Here's the drawing with two shaded views (mm, measured from the low corner). I have some questions. A direction names the side the tool comes from. Round coordinates to 2 decimals unless told otherwise and drop trailing zeros. Write each loop counter-clockwise with the first axis right and the second up, starting at its lowest first coordinate (ties: lowest second). Pieces come first, ordered by that corner, then holes. Notation, with made-up numbers: M 89,54.25 L 108,54.25 A19 cw 108,83.25 Z; hole C 73,3.5 d2. An arc over 180 degrees is marked long. Write item = value, one per line. Start each with the question number.
(1) I want a section at D-D (z = 4). Give the number of separate pieces and of enclosed holes in the cut face, and give its area (3 significant figures).
(2) I want a section at B-B (x = 69.85). List the corners of the cut face in (y, z) for me (1 decimal).
(3) Will these pins go through, and if not, where does the flat tip stop? pin 1 Ø1 at (y, z) = (9, 3) entering from +X; pin 2 Ø4.5 at (x, z) = (31.5, 1.5) entering from -Y (1 decimal); pin 3 Ø4.5 at (x, z) = (38, 2) entering from +Y (1 decimal); pin 4 Ø3 at (x, z) = (69.85, 8.89) entering from -Y.
(4) I need wall thicknesses on line 1 along Y through (x, z) = (25.4, 6.5); line 2 along X through (y, z) = (9.75, 8.75); line 3 along Y through (x, z) = (25.4, 4.25) (1 decimal). Which ranges of each line are inside material? Lowest first, please.
(5) I want a section at A-A (z = 8.89). List the corners of the cut face in (x, y) for me, and give its area (3 significant figures).
(6) On a 3-axis mill with a long thin cutter (end or side, diameter ignored), from which of +Z, -Z, +X, -X, +Y, -Y can I reach the whole of each face in a straight line? I mean the marked faces 1, 2 and 3. Say none if no direction works.
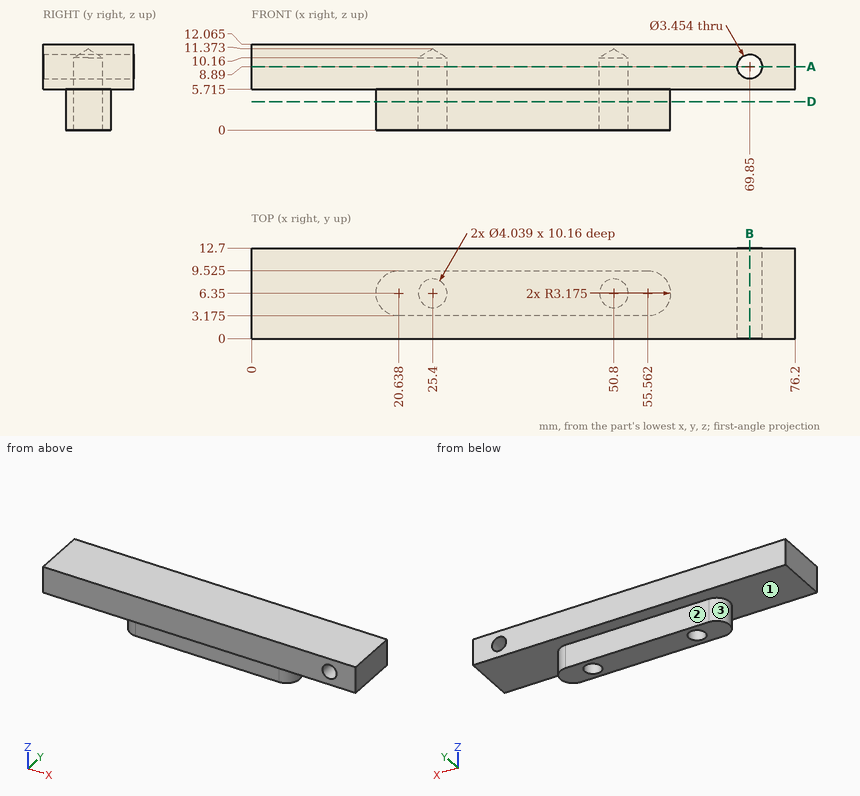
Returned:
q1.separate_pieces = 1
q1.enclosed_holes = 2
q1.area = 228 mm²
q2.outline = M 0,5.7 L 12.7,5.7 L 12.7,7.2 L 0,7.2 Z; M 0,10.6 L 12.7,10.6 L 12.7,12.1 L 0,12.1 Z
q3.pin_1 = 57.9
q3.pin_2 = 3.2
q3.pin_3 = 9.5
q3.pin_4 = through
q4.line_1 = 0 to 4.33, 8.37 to 12.7
q4.line_2 = 0 to 68.13, 71.57 to 76.2
q4.line_3 = 3.2 to 4.3, 8.4 to 9.5
q5.outline = M 0,0 L 68.12,0 L 68.12,12.7 L 0,12.7 Z; M 71.58,0 L 76.2,0 L 76.2,12.7 L 71.58,12.7 Z; hole C 25.4,6.35 d4.04; hole C 50.8,6.35 d4.04
q5.area = 898 mm²
q6.face_1 = -Z
q6.face_2 = -Z, +X, -X, +Y
q6.face_3 = -Z, -X
